Input: dimensioned drawing with shaded views. Units: mm. Origin: part minimum x, y, z. A direction names the side the tool comes from. Round coordinates to 2 decimals unless told otherwise and drop trailing zeros. Loops run counter-clockwise (first coordinate to the right, second up) from the corner with the lowest first, then second, coordinate; pieces in that order, holes last.
1) Section A-A, the plane y = 32.5. Return loops of the section in (x, z) (1 decimal), and give its area (3 significant figures).
2) First-contact query: pin 1 (12 mm diameter, centred on y = 95.5, z = 37, fed in from +X); pin 2 (1.5 mm diameter, centred on y = 85, z = 67.5, fed in from -X); pin 3 (3 mm diameter, centred on x = 12.5, z = 44, fed in from -Y); pin 4 (5 mm diameter, centred on x = 72, y = 100.5, fed in from -Z). Flat tips, straight axial feed; report the tip coordinate or a pass-through.
3) Ray query, line 1 along Z through (x, y) = (46, 169); line 2 along X through (y, z) = (173.5, 47) (1 decimal); line 3 along X through (y, z) = (93, 28) (1 decimal). Return the intervals inside material, ascending.
4) Section B-B, the plane y = 166. Return loops of the section in (x, z) (1 decimal).
5) Draft query along Y for the marked faces 1, 2, 3 and 4. Return one class per face: pulls with the +Y half, pulls with the -Y half, needs draft (parallel to the pull), parting line crosses it, or undercut.
6) Access query for the marked faces 5, 6 and 7. Directions: +Z, -Z, +X, -X, +Y, -Y. A direction counts if a zero-diameter tool reaches every point of the face in a straight line with its end or side. Return the directions, or none.
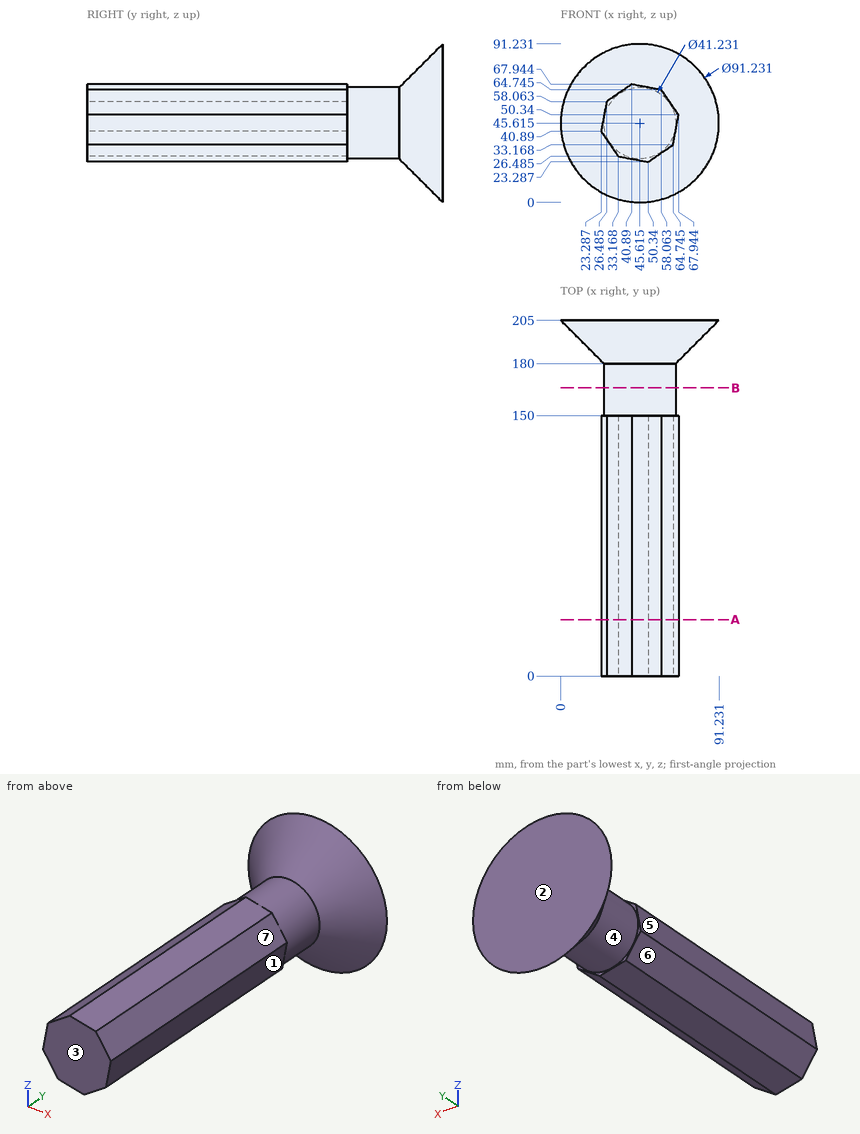
Final values:
1. outline: (23.3, 40.9) - (33.2, 26.5) - (50.3, 23.3) - (64.7, 33.2) - (67.9, 50.3) - (58.1, 64.7) - (40.9, 67.9) - (26.5, 58.1) - close
1. area: 1,470 mm2
2. pin 1: stops at x = 66.58
2. pin 2: stops at x = 39.15
2. pin 3: stops at y = 191.04
2. pin 4: passes through
3. line 1: z = 25 to 66.23
3. line 2: x = 25 to 66.2
3. line 3: x = 32.1 to 57.2
4. outline: circle Ø41.2 at (45.6, 45.6)
5. face 1: needs draft
5. face 2: pulls with the +Y half
5. face 3: pulls with the -Y half
5. face 4: undercut
6. face 5: +Z, -X, -Y
6. face 6: -Z, -X, -Y
6. face 7: +Z, +X, -Y
